Build history of the part. All positions in model axes, mm. Face numbers are marked on the shaded views. A direction names the side the tool comes from. Coordinates: 2 decimals unless noted, no trailing zeros. Write each loop counter-clockwise with the first axis right and the second up, starting at its lowest first coordinate (ties: lowest second). Pieces come first, ordered by that corner, then holes.
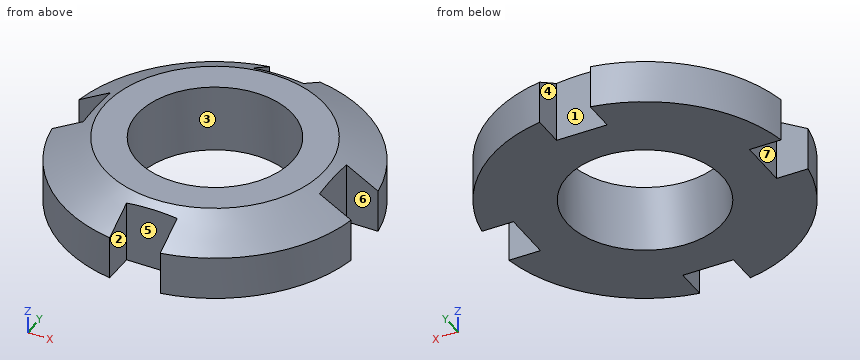
from build123d import *

# Parameters (mm, degrees)
TAP1_D             = 9.188
SKETCH4_W          = 3
SKETCH4_H          = 2
SKETCH4_W_2        = 2
SKETCH4_H_2        = 3
CUT_EXTRUDE1_DEPTH = 14.341664064


with BuildPart() as part:
    # Sketch1 → Revolve1 (revolve)
    with BuildSketch(Plane(origin=(0, 0, 0), x_dir=(0, 0, -1), z_dir=(1, 0, 0))):
        Polygon((0, 9), (-2.556624327, 9), (-4, 6.5), (-4, 0), (0, 0), align=None)
    revolve(axis=Axis((0, 0, 0), (0, 0, 1)))

    # Tap1 (through all)
    with Locations(Plane(origin=(0, 0, 0), x_dir=(-1, 0, 0), z_dir=(0, 0, -1))):
        with Locations((0, 0)):
            Hole(TAP1_D / 2)

    # Sketch4 → Cut-Extrude1 (cut, through all)
    with BuildSketch(Plane.XY):
        with Locations((0, 8)):
            Rectangle(SKETCH4_W, SKETCH4_H)
        with Locations((-8, 0)):
            Rectangle(SKETCH4_W_2, SKETCH4_H_2)
        with Locations((8, 0)):
            Rectangle(SKETCH4_W_2, SKETCH4_H_2)
        with Locations((0, -8)):
            Rectangle(SKETCH4_W, SKETCH4_H)
    extrude(amount=CUT_EXTRUDE1_DEPTH, mode=Mode.SUBTRACT)


solid = part.part
(1) Slice it at A-A, the plane x = 0. List the corners of the cut face in (y, z).
(2) Flat gauge pins, fed straight in: P1, Ø0.9, axis at y = -8, z = 1, coming from the -X side; P2, Ø0.9, axis at y = -8, z = 2, coming from the +X side; P3, Ø1.5, axis at y = 7.5, z = 2, coming from the +X side. Where does each tip first touch, or does it go through?
(3) Slice it at C-C, the plane z = 0.7. List the corners of the cut face in (x, y).
(4) Two-plate mould, pull along Y, no slides. Class the marked faces 1, 2 and 3: pulls with the +Y half, pulls with the -Y half, needs draft (parallel to the pull), parting line crosses it, or undercut.
(5) 3-axis set-ups, long thin cutter, end or side, ignore diameter. For the marked faces 4, 5, 6 and 7: which of +Z, -Z, +X, -X, +Y, -Y reach the whole face in a straight line?
(6) Probe L1, parallel to Y at x = 0, z = 1.2; L2, parallel to Y at x = -2.25, z = 2.8; L3, parallel to X at y = 2.5, z = 1.6. List the from-to ranges inside material, lowest first.
Results:
1. outline: (-7, 0) - (-4.59, 0) - (-4.59, 4) - (-6.5, 4) - (-7, 3.71) - close; (4.59, 0) - (7, 0) - (7, 3.71) - (6.5, 4) - (4.59, 4) - close
2. P1: stops at x = -4.9
2. P2: stops at x = 4.9
2. P3: stops at x = 5.95
3. outline: (-8.87, -1.5) arc R9 ccw to (-1.5, -8.87) - (-1.5, -7) - (1.5, -7) - (1.5, -8.87) arc R9 ccw to (8.87, -1.5) - (7, -1.5) - (7, 1.5) - (8.87, 1.5) arc R9 ccw to (1.5, 8.87) - (1.5, 7) - (-1.5, 7) - (-1.5, 8.87) arc R9 ccw to (-8.87, 1.5) - (-7, 1.5) - (-7, -1.5) - close; hole circle Ø9.19 at (0, 0)
4. face 1: pulls with the +Y half
4. face 2: needs draft
4. face 3: undercut
5. face 4: +Z, -Z, +Y
5. face 5: +Z, -Z, -Y
5. face 6: +Z, -Z, +X
5. face 7: +Z, -Z, -X
6. L1: y = -7 to -4.59, 4.59 to 7
6. L2: y = -8.28 to -4.01, 4.01 to 8.28
6. L3: x = -8.65 to -3.85, 3.85 to 8.65
